```python
from build123d import *

# Parameters (mm, degrees)
SKETCH1_R           = 1.35
SKETCH1_R_2         = 1.3
BOSS_EXTRUDE1_DEPTH = 7.5
CUT_EXTRUDE1_DEPTH  = 3.6
CHAMFER1_SIZE       = 1.5
SKETCH3_W           = 85
SKETCH3_H           = 2
CUT_EXTRUDE2_DEPTH  = 2.2
CUT_EXTRUDE3_REACH  = 9.5
SKETCH4_R           = 1.5


with BuildPart() as part:
    # Sketch1 → Boss-Extrude1 (new body)
    with BuildSketch(Plane.XY):
        with BuildLine():
            Line((42.5, -25), (42.5, 25))
            ThreePointArc((42.5, 25), (41.621320344, 27.121320344), (39.5, 28))
            Line((39.5, 28), (-39.5, 28))
            ThreePointArc((-39.5, 28), (-41.621320344, 27.121320344), (-42.5, 25))
            Line((-42.5, 25), (-42.5, -25))
            ThreePointArc((-42.5, -25), (-41.621320344, -27.121320344), (-39.5, -28))
            Line((-39.5, -28), (39.5, -28))
            ThreePointArc((39.5, -28), (41.621320344, -27.121320344), (42.5, -25))
        make_face()
        with Locations((-19, -24.5)):
            Circle(SKETCH1_R, mode=Mode.SUBTRACT)
        with Locations((39, -24.5)):
            Circle(SKETCH1_R, mode=Mode.SUBTRACT)
        with Locations((39, 24.5)):
            Circle(SKETCH1_R_2, mode=Mode.SUBTRACT)
        with Locations((-19, 24.5)):
            Circle(SKETCH1_R, mode=Mode.SUBTRACT)
    extrude(amount=BOSS_EXTRUDE1_DEPTH)

    # Sketch2 → Cut-Extrude1 (cut)
    with BuildSketch(Plane(origin=(0, 0, 0), x_dir=(-1, 0, 0), z_dir=(0, 0, -1))):
        with BuildLine():
            Line((15.5, 28), (-35.5, 28))
            Line((-35.5, 28), (-35.5, 21))
            Line((-35.5, 21), (-42.5, 21))
            Line((-42.5, 21), (-42.5, -21))
            Line((-42.5, -21), (-35.5, -21))
            Line((-35.5, -21), (-35.5, -28))
            Line((-35.5, -28), (15.5, -28))
            Line((15.5, -28), (15.5, -21))
            Line((15.5, -21), (22.5, -21))
            Line((22.5, -21), (22.5, -28))
            Line((22.5, -28), (39.5, -28))
            ThreePointArc((39.5, -28), (41.621320344, -27.121320344), (42.5, -25))
            Line((42.5, -25), (42.5, 25))
            ThreePointArc((42.5, 25), (41.621320344, 27.121320344), (39.5, 28))
            Line((39.5, 28), (22.5, 28))
            Line((22.5, 28), (22.5, 21))
            Line((22.5, 21), (15.5, 21))
            Line((15.5, 21), (15.5, 28))
        make_face()
    extrude(amount=-CUT_EXTRUDE1_DEPTH, mode=Mode.SUBTRACT)

    # Chamfer1
    chamfer1_edges = [part.edges().sort_by_distance(p)[0] for p in [
        (41.621320344, 27.121320344, 7.5),
        (0, 28, 7.5),
        (-41.621320344, 27.121320344, 7.5),
        (-42.5, 0, 7.5),
        (-41.621320344, -27.121320344, 7.5),
        (0, -28, 7.5),
        (41.621320344, -27.121320344, 7.5),
        (42.5, 0, 7.5),
    ]]
    chamfer(chamfer1_edges, length=CHAMFER1_SIZE)

    # Sketch3 → Cut-Extrude2 (cut)
    with BuildSketch(Plane.XY.offset(7.5)):
        with Locations((0, 20)):
            Rectangle(SKETCH3_W, SKETCH3_H)
        with Locations((0, 16)):
            Rectangle(SKETCH3_W, SKETCH3_H)
        with Locations((0, 12)):
            Rectangle(SKETCH3_W, SKETCH3_H)
        with Locations((0, 8)):
            Rectangle(SKETCH3_W, SKETCH3_H)
        with Locations((0, 4)):
            Rectangle(SKETCH3_W, SKETCH3_H)
        Rectangle(SKETCH3_W, SKETCH3_H)
        with Locations((0, -4)):
            Rectangle(SKETCH3_W, SKETCH3_H)
        with Locations((0, -8)):
            Rectangle(SKETCH3_W, SKETCH3_H)
        with Locations((0, -12)):
            Rectangle(SKETCH3_W, SKETCH3_H)
        with Locations((0, -16)):
            Rectangle(SKETCH3_W, SKETCH3_H)
        with Locations((0, -20)):
            Rectangle(SKETCH3_W, SKETCH3_H)
    extrude(amount=-CUT_EXTRUDE2_DEPTH, mode=Mode.SUBTRACT)

    # Sketch4 → Cut-Extrude3 (cut, up to next)
    with BuildSketch(Plane.XY.offset(7.5), mode=Mode.PRIVATE) as cut_extrude3_sk1:
        with Locations((-26.3, 24.5)):
            Circle(SKETCH4_R)
    cut_extrude3_tool1 = extrude(cut_extrude3_sk1.sketch, amount=-CUT_EXTRUDE3_REACH, mode=Mode.PRIVATE) & part.part
    add(cut_extrude3_tool1.solids().sort_by_distance((-26.3, 24.5, 7.5))[0], mode=Mode.SUBTRACT)
    # Sketch4 → Cut-Extrude3 (cut, up to next)
    with BuildSketch(Plane.XY.offset(7.5), mode=Mode.PRIVATE) as cut_extrude3_sk2:
        with Locations((31.7, 24.5)):
            Circle(SKETCH4_R)
    cut_extrude3_tool2 = extrude(cut_extrude3_sk2.sketch, amount=-CUT_EXTRUDE3_REACH, mode=Mode.PRIVATE) & part.part
    add(cut_extrude3_tool2.solids().sort_by_distance((31.7, 24.5, 7.5))[0], mode=Mode.SUBTRACT)
    # Sketch4 → Cut-Extrude3 (cut, up to next)
    with BuildSketch(Plane.XY.offset(7.5), mode=Mode.PRIVATE) as cut_extrude3_sk3:
        with Locations((-26.3, -24.5)):
            Circle(SKETCH4_R)
    cut_extrude3_tool3 = extrude(cut_extrude3_sk3.sketch, amount=-CUT_EXTRUDE3_REACH, mode=Mode.PRIVATE) & part.part
    add(cut_extrude3_tool3.solids().sort_by_distance((-26.3, -24.5, 7.5))[0], mode=Mode.SUBTRACT)
    # Sketch4 → Cut-Extrude3 (cut, up to next)
    with BuildSketch(Plane.XY.offset(7.5), mode=Mode.PRIVATE) as cut_extrude3_sk4:
        with Locations((31.7, -24.5)):
            Circle(SKETCH4_R)
    cut_extrude3_tool4 = extrude(cut_extrude3_sk4.sketch, amount=-CUT_EXTRUDE3_REACH, mode=Mode.PRIVATE) & part.part
    add(cut_extrude3_tool4.solids().sort_by_distance((31.7, -24.5, 7.5))[0], mode=Mode.SUBTRACT)


solid = part.part
```
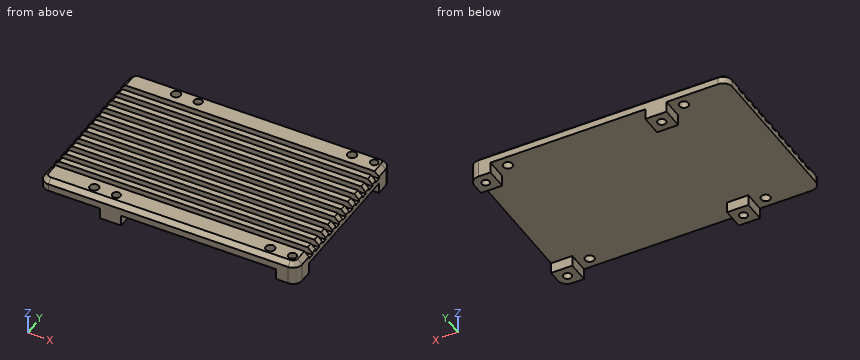
Input: part model. Units: mm. Frame: model coordinates. Coordinates: 2 decimals unless noted, no trailing zeros. Write each loop counter-clockwise with the first axis right and the second up, starting at its lowest first coordinate (ties: lowest second). Pieces come first, ordered by that corner, then holes.
1) Section D-D on y = -12. Output: boundary loops of the cut face in (x, z), and give its area (4 significant figures).
2) Material intervals for line 1 along Y through (x, z) = (-19, 2.25); line 2 along Y through (x, z) = (-26.3, 5); line 3 along Y through (x, z) = (37.5, 2.5), sorted ascending.
3) Pin query (flat end, axial travel): pin 1 Ø3.5 at (x, y) = (31.7, -24.5) entering from -Z; pin 2 Ø0.6 at (x, y) = (-8.5, -4) entering from +Z. Return the tip coordinate at first contact, or that it passes through.
4) Section B-B on y = 6. Output: boundary loops of the cut face in (x, z).
5) Section C-C on x = 31.7. State how many separate pieces and enclosed holes the cut face has, and give its area (3 significant figures).
6) Section A-A on z = 2.25. Output: boundary loops of the cut face in (x, y), and give its area (3 significant figures).
Check result:
1. outline: (-42.5, 3.6) - (42.5, 3.6) - (42.5, 5.3) - (-42.5, 5.3) - close
1. area: 144.5 mm2
2. line 1: y = -28 to -25.85, -23.15 to -21, 21 to 23.15, 25.85 to 28
2. line 2: y = -28 to -26, -23 to 23, 26 to 28
2. line 3: y = -28 to -21, 21 to 28
3. pin 1: stops at z = 3.6
3. pin 2: stops at z = 5.3
4. outline: (-42.5, 3.6) - (42.5, 3.6) - (42.5, 6) - (41, 7.5) - (-41, 7.5) - (-42.5, 6) - close
5. separate pieces: 3
5. enclosed holes: 0
5. area: 144 mm2
6. outline: (-22.5, -28) - (-15.5, -28) - (-15.5, -21) - (-22.5, -21) - close; (-22.5, 21) - (-15.5, 21) - (-15.5, 28) - (-22.5, 28) - close; (35.5, -28) - (39.5, -28) arc R3 ccw to (42.5, -25) - (42.5, -21) - (35.5, -21) - close; (35.5, 21) - (42.5, 21) - (42.5, 25) arc R3 ccw to (39.5, 28) - (35.5, 28) - close; hole circle Ø2.7 at (-19, -24.5); hole circle Ø2.7 at (-19, 24.5); hole circle Ø2.7 at (39, -24.5); hole circle Ø2.6 at (39, 24.5)
6. area: 170 mm2
